Input: part model. Units: mm. Frame: model coordinates. Face numbers are marked on the shaded views. Coordinates: 2 decimals unless noted, no trailing zeros. Order: outer loops, then holes, each group sorted by start corner. A loop starts at its lowest first (then second) coordinate and runs counter-clockwise, first axis right, second up.
from build123d import *

# Parameters (mm, degrees)
M25X1_5_TAPPED_HOLE2_D     = 23.5
FILLET1_R                  = 8
M10X1_0_TAPPED_HOLE1_D     = 9
M10X1_0_TAPPED_HOLE1_DEPTH = 10
M10X1_0_TAPPED_HOLE1_TIP   = 2.703872786


with BuildPart() as part:
    # Sketch1 → Revolve1 (revolve)
    with BuildSketch(Plane.XY, mode=Mode.PRIVATE) as revolve1_sk:
        Polygon((0, 12.478494624), (22, 12.478494624), (31, -13.521505376), (31, -33.521505376), (0, -33.521505376), align=None)
    revolve(revolve1_sk.sketch.rotate(Axis((0, 17.682795699, 0), (0, -1, 0)), 90), axis=Axis((0, 17.682795699, 0), (0, -1, 0)))

    # M25x1.5 Tapped Hole2 (through all)
    with Locations(Plane(origin=(0, 12.478494624, 0), x_dir=(1, 0, 0), z_dir=(0, 1, 0))):
        with Locations((0, 0)):
            Hole(M25X1_5_TAPPED_HOLE2_D / 2)

    # Fillet1
    fillet1_edges = [part.edges().sort_by_distance(p)[0] for p in [
        (0, 12.478494624, -22),
    ]]
    fillet(fillet1_edges, radius=FILLET1_R)

    # M10x1.0 Tapped Hole1
    with Locations(Plane(origin=(0, 8.13574381, 23.503259897), x_dir=(1, 0, 0), z_dir=(0, 0.32711056388316645, 0.9449860734402581))):
        with Locations((0, -11.100931225)):
            Hole(M10X1_0_TAPPED_HOLE1_D / 2, depth=M10X1_0_TAPPED_HOLE1_DEPTH)
            with Locations((0, 0, -(M10X1_0_TAPPED_HOLE1_DEPTH + M10X1_0_TAPPED_HOLE1_TIP / 2))):  # 118° drill point
                Cone(0, M10X1_0_TAPPED_HOLE1_D / 2, M10X1_0_TAPPED_HOLE1_TIP, mode=Mode.SUBTRACT)


solid = part.part
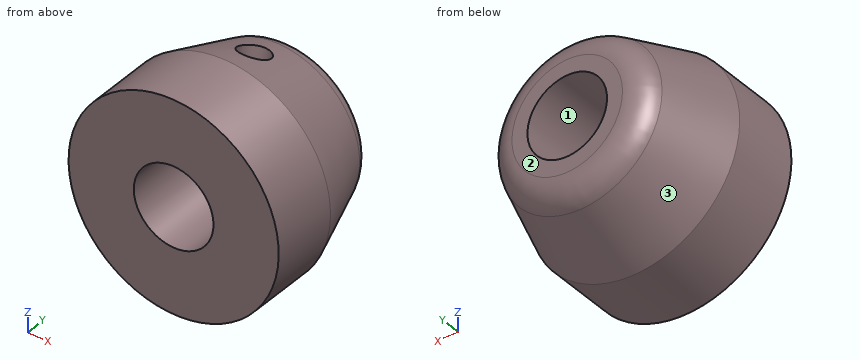
Item 1: Draft query along X for the marked faces 1, 2 and 3. Return one class per face: pulls with the +X half, pulls with the -X half, needs draft (parallel to the pull), parting line crosses it, or undercut.
Response values:
face 1: undercut
face 2: needs draft
face 3: parting line crosses it
Item 2: Cut plane C-C on y = -8. Count the separate pieces of the cut face and the enclosed holes in it, then the cut area to 3 significant figures.
Response values:
separate pieces: 1
enclosed holes: 2
area: 2,190 mm2
Item 3: Cut plane B-B on y = -15. Return loops of the section in (x, z).
Response values:
outline: circle Ø62 at (0, 0); hole circle Ø23.5 at (0, 0)
Item 4: Cut plane A-A on z = 0. Return loops of the section in (x, y).
Response values:
outline: (-31, -33.52) - (-11.75, -33.52) - (-11.75, 12.48) - (-16.3, 12.48) arc R8 ccw to (-23.86, 7.1) - (-31, -13.52) - close; (11.75, -33.52) - (31, -33.52) - (31, -13.52) - (23.86, 7.1) arc R8 ccw to (16.3, 12.48) - (11.75, 12.48) - close
Item 5: Ray query, probe 1 along X at (y, z) = (-20.5, -6.5); probe 2 along X at (y, z) = (1.5, 10); probe 3 along Z at (x, y) = (0, -4). Return the intervals inside material, ascending.
Response values:
probe 1: x = -30.31 to -9.79, 9.79 to 30.31
probe 2: x = -23.78 to -6.17, 6.17 to 23.78
probe 3: z = -27.7 to -11.75, 11.75 to 15.66
Item 6: Pin query (flat end, axial travel): pin 1 Ø5 at (y, z) = (-14.5, -14.5) entering from -X; pin 2 Ø5 at (y, z) = (-22, -1.5) entering from +X; pin 3 Ø12 at (y, z) = (6, 13.5) entering from -X. Return the tip coordinate at first contact, or that it passes through.
Response values:
pin 1: stops at x = -28.58
pin 2: stops at x = 31
pin 3: stops at x = -23.99
